Read the model definition and answer for the solid it produces. Units are mm, in the model's axes. A direction names the side the tool comes from. Give positions to 0.01 mm unless a question says otherwise; leave off trailing zeros. Order: outer loops, then holes, each group sorted by start corner. A loop starts at its lowest first (then second) coordinate and runs counter-clockwise, first axis right, second up. Notation, with made-up numbers: (50, 80) - (74, 80) arc R18 ccw to (74, 100) - close; hole circle Ø8 at (-28.5, 33). An arc over 180 degrees is marked (long way). Write item = value, one per line.
Autodesk Inventor part; units mm, degrees
ref_plane "YZ Plane" through (0, 0, 0) normal (1, 0, 0) x (0, 1, 0)
ref_plane "XZ Plane" through (0, 0, 0) normal (0, 1, 0) x (-1, 0, 0)
ref_plane "XY Plane" through (0, 0, 0) normal (0, 0, 1) x (1, 0, 0)
sketch "Sketch1" plane through (0, 0, 0) normal (0, 0, 1) x (1, 0, 0)
  line L0 (0, 0) -> (-25.4, 0)
  line L1 (-25.4, 0) -> (-25.4, 38.735)
  line L2 (-25.4, 38.735) -> (0, 38.735)
  line L3 (0, 38.735) -> (0, 0)
  dimension "d0" = 25.4
  dimension "d1" = 38.735
extrude "Extrusion1" add sketch "Sketch1" along normal blind 7.62
sketch "Sketch5" plane through (0, 0, 7.62) normal (0, 0, 1) x (1, 0, 0)
  line L0 (-25.4, 0) -> (0, 0)
  line L1 (-25.4, 38.735) -> (-25.4, 0)
  line L2 (0, 0) -> (-25.4, 0)
  line L3 (-25.4, 0) -> (-25.4, 5.08)
  line L4 (-25.4, 5.08) -> (0, 5.08)
  line L5 (0, 5.08) -> (0, 0)
  line L6 (0, 38.735) -> (-25.4, 38.735)
  line L7 (-25.4, 38.735) -> (-25.4, 33.655)
  line L8 (-25.4, 33.655) -> (0, 33.655)
  line L9 (0, 33.655) -> (0, 38.735)
  line L10 (0, 38.735) -> (-25.4, 38.735)
  dimension "d29" = 5.08
  dimension "d30" = 5.08
  dimension "d31" = 0
extrude "Extrusion4" add sketch "Sketch5" along normal blind 28.575
sketch "Sketch6" plane through (0, 0, 36.195) normal (0, 0, 1) x (1, 0, 0)
  line L0 (-25.4, 0) -> (-25.4, 38.735)
  line L1 (-25.4, 38.735) -> (0, 38.735)
  line L2 (0, 38.735) -> (0, 32.385)
  line L3 (0, 32.385) -> (-25.4, 32.385)
  line L4 (-25.4, 32.385) -> (-25.4, 38.735)
  line L5 (-25.4, 0) -> (0, 0)
  line L6 (0, 0) -> (0, 6.35)
  line L7 (0, 6.35) -> (-25.4, 6.35)
  line L8 (-25.4, 6.35) -> (-25.4, 0)
  line L9 (-25.4, 33.655) -> (0, 33.655)
  dimension "d34" = 5.08
  dimension "d35" = 6.35
  dimension "d36" = 6.35
  dimension "d37" = 25.4
  dimension "d38" = 25.4
extrude "Extrusion5" add sketch "Sketch6" along normal blind 2.54
sketch "Sketch7" plane through (0, 0, 7.62) normal (0, 0, 1) x (1, 0, 0)
  line L0 (-25.4, 33.655) -> (-25.4, 5.08)
  line L1 (-25.4, 32.385) -> (0, 32.385)
  line L2 (0, 32.385) -> (0, 6.35)
  line L3 (0, 6.35) -> (-25.4, 6.35)
  line L4 (-25.4, 6.35) -> (-25.4, 32.385)
  line L5 (-25.4, 5.08) -> (0, 5.08)
  point P0 (0, 0)
  dimension "d41" = 26.035
  dimension "d42" = 1.27
  dimension "d43" = 25.4
extrude "Extrusion6" cut sketch "Sketch7" against normal blind 2.54
fillet "Fillet2" radius 3.175 4 edges at (0, 33.655, 21.9075) (-25.4, 33.655, 21.9075) (-25.4, 5.08, 21.9075) (0, 5.08, 21.9075)
sketch "Sketch8" plane through (0, 0, 0) normal (0, 0, -1) x (-1, 0, 0)
  line L0 (25.4, 0) -> (25.4, 38.735)
  line L1 (0, 38.735) -> (0, 0)
  line L2 (25.4, 38.735) -> (0, 38.735)
  line L3 (0, 0) -> (25.4, 0)
  point P0 (12.7, 19.3675)
  dimension "d47" = 12.7
  dimension "d48" = 25.4
  dimension "d49" = 38.735
  dimension "d50" = 19.3675
hole "Hole2" at (-12.7, 19.3675, 0) direction (0, 0, 1) diameter 4.4958 end through all
equation "\"d30\" = d29"
equation "\"d36\" = d35"
properties part number "chain tensioner"
1. Flat-ended cylindrical pins translate along their axes: pin 1 (2.5 mm diameter, centred on x = -12.7, y = 19.37, fed in from +Z); pin 2 (5.5 mm diameter, centred on x = -17.5, z = 26.5, fed in from -Y); pin 3 (7.5 mm diameter, centred on x = -13, y = 18.5, fed in from +Z). Find the tip coordinate at first contact, or state that the pin passes through.
Recorded:
pin_1 = through
pin_2 = 0
pin_3 = 5.08
2. Section B-B (x = -12.7) is taken. Determine the outline of the cut face in (y, z) (3 decimals), and give its area (3 significant figures).
Recorded:
outline = (0, 0) - (17.12, 0) - (17.12, 5.08) - (6.35, 5.08) - (6.35, 7.62) - (5.08, 7.62) - (5.08, 36.195) - (6.35, 36.195) - (6.35, 38.735) - (0, 38.735) - close; (21.615, 0) - (38.735, 0) - (38.735, 38.735) - (32.385, 38.735) - (32.385, 36.195) - (33.655, 36.195) - (33.655, 7.62) - (32.385, 7.62) - (32.385, 5.08) - (21.615, 5.08) - close
area = 529 mm^2
3. Section D-D (y = 18) is taken. Determine the outline of the cut face in (x, z), and give its area (3 significant figures).
Recorded:
outline = (-25.4, 0) - (-14.48, 0) - (-14.48, 5.08) - (-25.4, 5.08) - close; (-10.92, 0) - (0, 0) - (0, 5.08) - (-10.92, 5.08) - close
area = 111 mm^2
4. Section A-A (z = 19.5) is taken. Determine the outline of the cut face in (x, y) (3 decimals), and give its area (3 significant figures).
Recorded:
outline = (-25.4, 0) - (0, 0) - (0, 1.905) arc R3.175 ccw to (-3.175, 5.08) - (-22.225, 5.08) arc R3.175 ccw to (-25.4, 1.905) - close; (-25.4, 36.83) arc R3.175 ccw to (-22.225, 33.655) - (-3.175, 33.655) arc R3.175 ccw to (0, 36.83) - (0, 38.735) - (-25.4, 38.735) - close
area = 249 mm^2
5. For faces 1 (the face through (-25.4, 19.3, 4.9)), 2 (the face through (-24.495, 34.61, 22.108)), 3 (the face through (-0.955, 34.56, 22.108)), 4 (the face through (-13, 33.655, 22)), 5 (the face through (-13, 32.385, 37)), determine the directions among +Z, -Z, +X, -X, +Y, -Y from which every point of the face is accessible in a straight line to the end or side of a thin tool.
Recorded:
face_1 = +Z, -Z, -X, +Y, -Y
face_2 = -X
face_3 = +X
face_4 = +X, -X
face_5 = +Z, +X, -X
6. Section C-C (z = 4.5) is taken. Determine the outline of the cut face in (x, y) (1 decimal), and give its area (3 significant figures).
Recorded:
outline = (-25.4, 0) - (0, 0) - (0, 38.7) - (-25.4, 38.7) - close; hole circle Ø4.5 at (-12.7, 19.4)
area = 968 mm^2
7. Straight lines are drawn through the part: L1, parallel to Y at x = -12.7, z = 4 (3 decimals); L2, parallel to Y at x = -4.25, z = 7.5 (3 decimals); L3, parallel to Z at x = -20.5, y = 27.5. For each, find the intervals that lie inside material, in ascending order. Write a range as [from, to].
Recorded:
L1 = [0, 17.12], [21.615, 38.735]
L2 = [0, 6.35], [32.385, 38.735]
L3 = [0, 5.08]
8. Determine the mould class of faces 6 (the face through (-13, 0, 19)), 7 (the face through (-13, 38.735, 19)), 8 (the face through (-13, 32.385, 6)), 9 (the face through (0, 19.5, 4.9)) for opening direction Y: +Y half, -Y half, draft (parallel to the pull), parting line (faces both ways), or undercut.
Recorded:
face_6 = -Y half
face_7 = +Y half
face_8 = undercut
face_9 = draft
